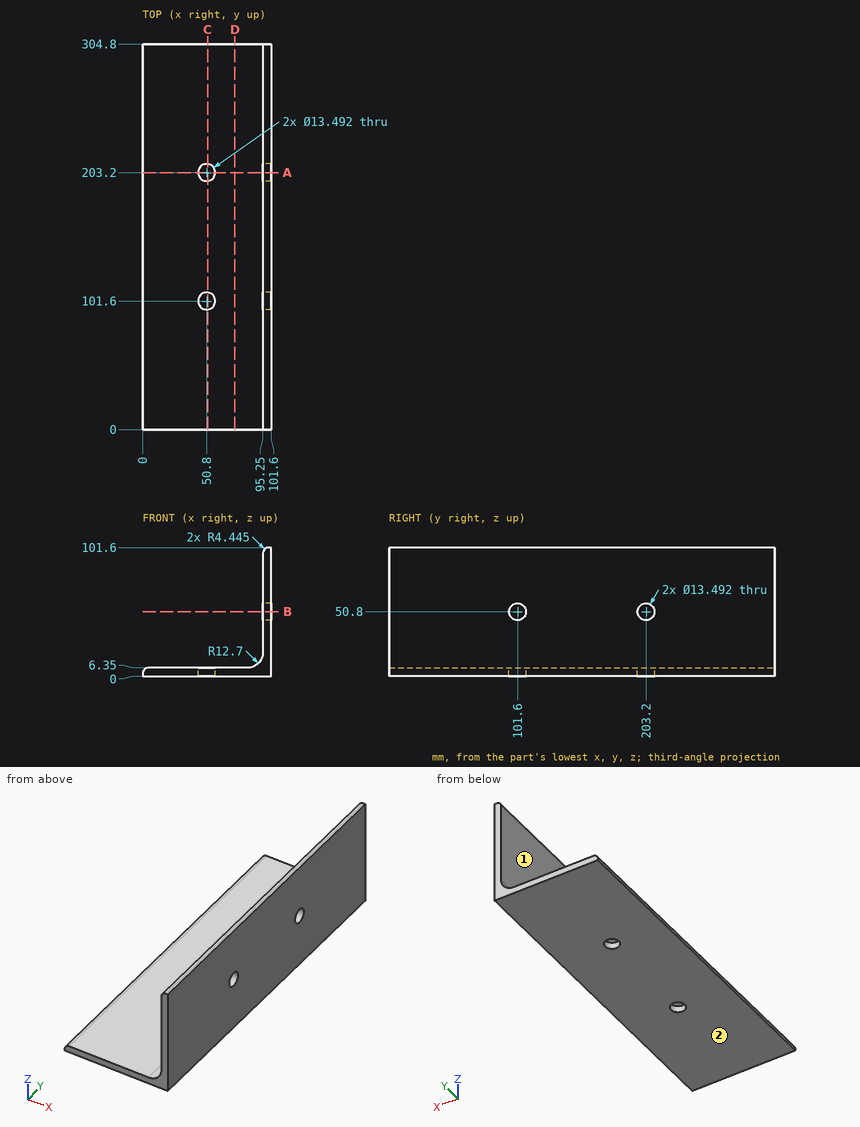
For this review, use the dimensioned drawing (mm, ordinates from the lowest corner) and the shaded views. A direction names the side the tool comes from. Round coordinates to 2 decimals unless told otherwise and drop trailing zeros. Order: outer loops, then holes, each group sorted by start corner. A loop starts at its lowest first (then second) coordinate and runs counter-clockwise, first axis right, second up. Notation, with made-up numbers: M 89.5,-28 L 145.5,-28 A20 cw 145.5,-21 Z; hole C 28,2 d5. An arc over 180 degrees is marked long. Use a Markdown table: item, result. Add a question column.
Item 1: Add section D-D, the plane x = 73. Give the boundary of the cut face in (y, z).
Item 2: To check wall thickness, follow line 1 along Y through (x, z) = (50, 5); line 2 along Z through (x, y) = (99, 203) (1 decimal); line 3 along Z through (x, y) = (24.5, 243). State the ranges of each line that lie inside material, in increasing order.
Item 3: Add section C-C, the plane x = 51.5. Give the boundary of the cut face in (y, z).
Item 4: Add section B-B, the plane z = 50.8. Give the boundary of the cut face in (x, y), then the cut area to 3 significant figures.
Item 5: Add section A-A, the plane y = 203.2. State how many separate pieces and enclosed holes the cut face has.
Item 6: Insertion check: pin 1 (12 mm diameter, centred on y = 78, z = 34, fed in from -X); pin 2 (15.5 mm diameter, centred on x = 50.8, y = 203.2, fed in from +Z). Each pin has a flat end and moves straight along its axis. Give the tip position at first contact, or say it passes through.
Item 7: Tool access review of the marked faces 1 and 2: name each direction out of +Z, -Z, +X, -X, +Y, -Y from which nothing blocks a thin tool from reaching the whole face with its end or side.
Geometry results:
| question | item | result |
|---|---|---|
| 1 | outline | M 0,0 L 304.8,0 L 304.8,6.35 L 0,6.35 Z |
| 2 | line 1 | y = 0 to 94.9, 108.3 to 196.5, 209.9 to 304.8 |
| 2 | line 2 | z = 0 to 44.1, 57.5 to 101.5 |
| 2 | line 3 | z = 0 to 6.35 |
| 3 | outline | M 0,0 L 94.89,0 L 94.89,6.35 L 0,6.35 Z; M 108.31,0 L 196.49,0 L 196.49,6.35 L 108.31,6.35 Z; M 209.91,0 L 304.8,0 L 304.8,6.35 L 209.91,6.35 Z |
| 4 | outline | M 95.25,0 L 101.6,0 L 101.6,94.85 L 95.25,94.85 Z; M 95.25,108.35 L 101.6,108.35 L 101.6,196.45 L 95.25,196.45 Z; M 95.25,209.95 L 101.6,209.95 L 101.6,304.8 L 95.25,304.8 Z |
| 4 | area | 1,760 mm² |
| 5 | separate pieces | 3 |
| 5 | enclosed holes | 0 |
| 6 | pin 1 | stops at x = 95.25 |
| 6 | pin 2 | stops at z = 6.35 |
| 7 | face 1 | +Z, -X, +Y, -Y |
| 7 | face 2 | -Z, +X, -X, +Y, -Y |
